Check sheet for the modelled part. Datum: model origin and axes. Units: mm. Face numbers are marked on the shaded views. A direction names the side the tool comes from. Give positions to 0.01 mm unless a question says otherwise; leave off trailing zeros. Order: outer loops, then holes, each group sorted by start corner. A loop starts at its lowest first (then second) coordinate and runs counter-clockwise, first axis right, second up.
Item 1: Sectioned sample at A-A on x = 26.5. Record the boundary of the cut face in (y, z), and give its area (3 significant figures).
Item 2: Gauge pin test, flat ends, axial feed: P1, Ø8, axis at x = -8.5, y = 5.5, coming from the -Z side; P2, Ø6, axis at y = 7.5, z = 51.5, coming from the +X side; P3, Ø4.5, axis at x = 17.5, y = -12.5, coming from the +Z side; P4, Ø21, axis at x = 17.5, z = 23, coming from the -Y side. Record the tip position at first contact, or that the pin passes through.
Item 3: Sectioned sample at B-B on z = 13.5. Record the boundary of the cut face in (x, y), and give its area (3 significant figures).
Item 4: Material ranges on line 1 along Z through (x, y) = (9, -15.5); line 2 along X through (y, z) = (13, 31.5); line 3 along Y through (x, z) = (-19, 21), recorded low to high.
Item 5: Sectioned sample at C-C on y = 4.5. Record the boundary of the cut face in (x, z), and give its area (3 significant figures).
Item 6: Access from +Z, -Z, +X, -X, +Y, -Y to the whole of each face (thin tool, end or side, straight path). Record for the marked faces 1, 2, 3 and 4.
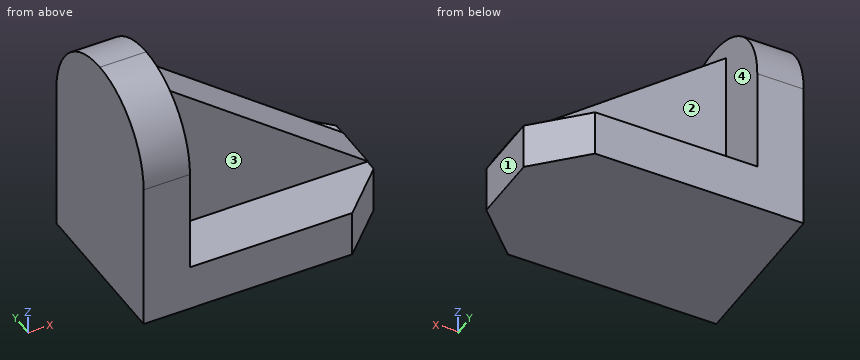
Autodesk Fusion 360 part; units mm, degrees
sketch "Sketch1" plane through (0, 0, 0) normal (0, 0, 1) x (1, 0, 0)
  line L0 (33, -21) -> (-33, -21)
  line L1 (-33, -21) -> (-33, 21)
  line L2 (-33, 21) -> (33, 21)
  line L3 (33, 21) -> (33, -21)
  line L4 (33, -21) -> (-33, 21) construction
  line L5 (-33, -21) -> (33, 21) construction
  dimension "d1" = 66
  dimension "d2" = 42
extrude "Extrude1" add sketch "Sketch1" along normal blind 12
chamfer "Chamfer1" distance 12 angle 45 2 edges at (33, -21, 6) (33, 21, 6)
sketch "Sketch2" plane through (0, 0, 12) normal (0, 0, 1) x (-1, 0, 0)
  line L0 (-33, -9) -> (-21, -21)
  line L1 (-21, -21) -> (33, -21)
  line L2 (33, -21) -> (33, 21)
  line L3 (33, 21) -> (-21, 21)
  line L4 (-21, 21) -> (-33, 9)
  line L5 (-33, 9) -> (-33, -9)
  line L6 (33, -21) -> (21, -21)
  line L7 (21, -21) -> (21, 21)
  line L8 (21, 21) -> (33, 21)
  line L9 (33, 21) -> (33, -21)
  dimension "d6" = 12
extrude "Extrude2" add sketch "Sketch2" along normal blind 48 contours L1 L2 L3 L6 L7 L8 L9
fillet "Fillet1" radius 21 2 edges at (-27, 21, 60) (-27, -21, 60)
sketch "Sketch3" plane through (0, 0, 0) normal (0, 1, 0) x (1, 0, 0)
  line L0 (-21, -12) -> (-21, -54)
  line L1 (-21, -54) -> (33.1488, -12)
  line L2 (33.1488, -12) -> (-21, -12)
  dimension "d11" = 42
extrude "Extrude3" add sketch "Sketch3" along normal mid plane 12
equation "d7 = 60.00 mm - 12.00 mm"
Report:
1. outline: (-15.5, 0) - (15.5, 0) - (15.5, 12) - (6, 12) - (6, 17.16) - (-6, 17.16) - (-6, 12) - (-15.5, 12) - close
1. area: 434 mm2
2. P1: stops at z = 0
2. P2: stops at x = -14.43
2. P3: stops at z = 12
2. P4: stops at y = -6
3. outline: (-33, -21) - (-21, -21) - (-21, -6) - (31.21, -6) - (31.21, 6) - (-21, 6) - (-21, 21) - (-33, 21) - close
3. area: 1,130 mm2
4. line 1: z = 0 to 12
4. line 2: x = -33 to -21
4. line 3: y = -6 to 6
5. outline: (-33, 0) - (33, 0) - (33, 12) - (33.15, 12) - (-21, 54) - (-21, 59.51) - (-33, 59.51) - close
5. area: 2,500 mm2
6. face 1: -Z, +X, +Y, -Y
6. face 2: +Z, +X, +Y
6. face 3: +Z, +X, -Y
6. face 4: +Z, +X
